```python
from build123d import *

# Parameters (mm, degrees)
F0_R     = 37
F1_DEPTH = 7
F2_R     = 4
F3_DEPTH = 21
F4_R     = 4
F5_DEPTH = 7
F6_R     = 6.5
F7_DEPTH = 14
F9_DEPTH = 28.001


with BuildPart() as f1:
    # F0 (on Top) → F1 (new body)
    with BuildSketch(Plane.XY):
        Circle(F0_R)
    extrude(amount=F1_DEPTH)

    # F2 (on face) → F3 (join)
    with BuildSketch(Plane(origin=(0, 0, 0), x_dir=(1, 0, 0), z_dir=(0, 0, -1))):
        Circle(F2_R)
    extrude(amount=F3_DEPTH)

    # F4 (on face) → F5 (join)
    with BuildSketch(Plane(origin=(0, 0, 0), x_dir=(1, 0, 0), z_dir=(0, 0, -1))):
        with Locations((-30, 0)):
            Circle(F4_R)
        with Locations((30, 0)):
            Circle(F4_R)
    extrude(amount=F5_DEPTH)

    # F6 (on face) → F7 (join)
    with BuildSketch(Plane(origin=(0, 0, 0), x_dir=(1, 0, 0), z_dir=(0, 0, -1))):
        Circle(F6_R)
    extrude(amount=F7_DEPTH)

    # F8 (on face) → F9 (cut, through all)
    with BuildSketch(Plane.XY.offset(7)):
        with BuildLine():
            Line((-4, -4), (-32.756679, -4))
            ThreePointArc((-32.756679, -4), (-23.334524, -23.334524), (-4, -32.756679))
            Line((-4, -32.756679), (-4, -4))
        make_face()
        with BuildLine():
            Line((-32.756679, 4), (-4, 4))
            Line((-4, 4), (-4, 32.756679))
            ThreePointArc((-4, 32.756679), (-23.334524, 23.334524), (-32.756679, 4))
        make_face()
        with BuildLine():
            Line((4, 4), (32.756679, 4))
            ThreePointArc((32.756679, 4), (23.334524, 23.334524), (4, 32.756679))
            Line((4, 32.756679), (4, 4))
        make_face()
        with BuildLine():
            Line((32.756679, -4), (4, -4))
            Line((4, -4), (4, -32.756679))
            ThreePointArc((4, -32.756679), (23.334524, -23.334524), (32.756679, -4))
        make_face()
    extrude(amount=-F9_DEPTH, mode=Mode.SUBTRACT)


solid = f1.part
```
Model file for the job. Use its own axes, mm. A direction names the side the tool comes from. Round coordinates to 2 decimals unless told otherwise and drop trailing zeros. Order: outer loops, then holes, each group sorted by start corner. A loop starts at its lowest first (then second) coordinate and runs counter-clockwise, first axis right, second up. Notation, with made-up numbers: (53.5, 23.25) -> (79.5, 23.25) arc R24 ccw to (79.5, 34.25) -> close; hole circle Ø8 at (6, -39.75). An arc over 180 degrees is marked (long way). Use one line per item in the form item = value.
Item 1: Cut at D-D, the plane y = 28. Write the cut outline in (x, z), and give its area (3 significant figures).
Returned:
outline = (-24.19, 0) -> (-17.46, 0) -> (-17.46, 7) -> (-24.19, 7) -> close; (-4, 0) -> (4, 0) -> (4, 7) -> (-4, 7) -> close; (17.46, 0) -> (24.19, 0) -> (24.19, 7) -> (17.46, 7) -> close
area = 150 mm^2
Item 2: Pull direction X, two halves, no side cores. Call faces 4 (the face through (0.1, -6.5, -6.9)), 5 (the face through (0, 0, -21)), 6 (the face through (23.117, -23.55, 3.549)), 7 (the face through (6.5, 0.1, -6.9)): released by +X, released by -X, zero draft, split by the parting line, or undercut.
Returned:
face_4 = split by the parting line
face_5 = zero draft
face_6 = undercut
face_7 = undercut
Item 3: Tool access for faces 1 (the face through (-30, 0, -7)), 2 (the face through (-6.5, -0.1, -6.9)), 3 (the face through (23.55, 23.117, 3.549)): list every direction of +Z, -Z, +X, -X, +Y, -Y with a clear straight run to the whole face (end or side of a thin tool).
Returned:
face_1 = -Z, -X, +Y, -Y
face_2 = -Z
face_3 = +Z, -Z
Item 4: Cut at A-A, the plane z = 4.5. Write the cut outline in (x, y), and give its area (3 significant figures).
Returned:
outline = circle Ø74 at (0, 0); hole (-32.76, -4) arc R33 ccw to (-4, -32.76) -> (-4, -4) -> close; hole (-32.76, 4) -> (-4, 4) -> (-4, 32.76) arc R33 ccw to start; hole (4, -32.76) arc R33 ccw to (32.76, -4) -> (4, -4) -> close; hole (4, 4) -> (32.76, 4) arc R33 ccw to (4, 32.76) -> close
area = 1,870 mm^2
Item 5: Drill centre lines: line 1 (Y direction, x = 18, z = 3.75); line 2 (X direction, y = -9, z = 4.75); line 3 (Y direction, x = -11, z = 5). Where is each one in solid material? Low to high.
Returned:
line_1 = -32.33 to -27.66, -4 to 4, 27.66 to 32.33
line_2 = -35.89 to -31.75, -4 to 4, 31.75 to 35.89
line_3 = -35.33 to -31.11, -4 to 4, 31.11 to 35.33
Item 6: Flat gauge pins, fed straight in: pin 1 Ø2.5 at (x, y) = (14.5, 1) entering from -Z; pin 2 Ø10.5 at (x, z) = (-12, 0) entering from +Y; pin 3 Ø10.5 at (x, z) = (-13.5, -4) entering from -Y. Where does each tip first touch, or does it go through?
Returned:
pin_1 = 0
pin_2 = 36.38
pin_3 = -35.59
Item 7: Cut at C-C, the plane z = -1.25. Write the cut outline in (x, y).
Returned:
outline = circle Ø8 at (-30, 0); (-5.12, -4) -> (-4, -4) -> (-4, -5.12) arc R6.5 ccw to (4, -5.12) -> (4, -4) -> (5.12, -4) arc R6.5 ccw to (5.12, 4) -> (4, 4) -> (4, 5.12) arc R6.5 ccw to (-4, 5.12) -> (-4, 4) -> (-5.12, 4) arc R6.5 ccw to start; circle Ø8 at (30, 0)
Item 8: Cut at B-B, the plane x = 0. Write the cut outline in (y, z), and give its area (3 significant figures).
Returned:
outline = (-37, 0) -> (-6.5, 0) -> (-6.5, -14) -> (-4, -14) -> (-4, -21) -> (4, -21) -> (4, -14) -> (6.5, -14) -> (6.5, 0) -> (37, 0) -> (37, 7) -> (-37, 7) -> close
area = 756 mm^2
